from build123d import *

# Parameters (mm, degrees)
SKETCH1_W           = 113.157
SKETCH1_H           = 113.157
SKETCH1_R           = 3.048
BOSS_EXTRUDE1_DEPTH = 8.73125
SKETCH1_3_W         = 113.157
SKETCH1_3_H         = 113.157
SKETCH1_3_R         = 3.33375
SKETCH1_3_R_2       = 50.8
SKETCH1_3_R_3       = 3.01625
SKETCH1_3_R_4       = 3.048
BOSS_EXTRUDE2_DEPTH = 9.525
SKETCH1_4_R         = 3.01625
BOSS_EXTRUDE3_DEPTH = 18.3515
CUT_EXTRUDE1_START  = -5.899214
SKETCH2_R           = 3.5
CUT_EXTRUDE1_DEPTH  = 5.899214
CIRPATTERN1_COUNT   = 4
SKETCH5_R           = 3.047999999
BOSS_EXTRUDE4_DEPTH = 9.525


with BuildPart() as part:
    # Sketch1 → Boss-Extrude1 (new body)
    with BuildSketch(Plane.XY):
        Rectangle(SKETCH1_W, SKETCH1_H)
        with Locations((-14.204320599, -16.928050104)):
            Circle(SKETCH1_R, mode=Mode.SUBTRACT)
    extrude(amount=BOSS_EXTRUDE1_DEPTH)

    # Sketch1<3> → Boss-Extrude2 (add)
    with BuildSketch(Plane.XY):
        Rectangle(SKETCH1_3_W, SKETCH1_3_H)
        with Locations((-43.8785, -43.8785)):
            Circle(SKETCH1_3_R, mode=Mode.SUBTRACT)
        with Locations((43.8785, -43.8785)):
            Circle(SKETCH1_3_R, mode=Mode.SUBTRACT)
        with Locations((43.8785, 43.8785)):
            Circle(SKETCH1_3_R, mode=Mode.SUBTRACT)
        with Locations((-43.8785, 43.8785)):
            Circle(SKETCH1_3_R, mode=Mode.SUBTRACT)
        Circle(SKETCH1_3_R_2, mode=Mode.SUBTRACT)
        with Locations((24.490207929, 29.186293283)):
            Circle(SKETCH1_3_R_3)
        with Locations((13.030967461, -35.802288852)):
            Circle(SKETCH1_3_R_3)
        Circle(SKETCH1_3_R_3)
        with Locations((-37.52117539, 6.615995569)):
            Circle(SKETCH1_3_R_3)
        with Locations((-14.204320599, -16.928050104)):
            Circle(SKETCH1_3_R_4)
    extrude(amount=-BOSS_EXTRUDE2_DEPTH)

    # Sketch1<4> → Boss-Extrude3 (add)
    with BuildSketch(Plane.XY):
        Circle(SKETCH1_4_R)
    extrude(amount=-BOSS_EXTRUDE3_DEPTH)

    # Sketch2 → Cut-Extrude1 (cut)
    with BuildSketch(Plane(origin=(0, 56.5785, 0), x_dir=(1, 0, 0), z_dir=(0, 1, 0)).offset(CUT_EXTRUDE1_START)):
        with Locations((0, 4.7625)):
            Circle(SKETCH2_R)
    cut_extrude1 = extrude(amount=CUT_EXTRUDE1_DEPTH, mode=Mode.SUBTRACT)

    # CirPattern1: Cut-Extrude1 ×4 about axis
    cirpattern1_axis = Axis((0, 0, -9.525), (0, 0, 1))
    for i in range(1, CIRPATTERN1_COUNT):
        add(cut_extrude1.rotate(cirpattern1_axis, i * 360 / CIRPATTERN1_COUNT), mode=Mode.SUBTRACT)

    # Sketch5 → Boss-Extrude4 (add)
    with BuildSketch(Plane.XY.offset(8.73125)):
        with Locations((-14.204320599, -16.928050104)):
            Circle(SKETCH5_R)
    extrude(amount=-BOSS_EXTRUDE4_DEPTH)


solid = part.part
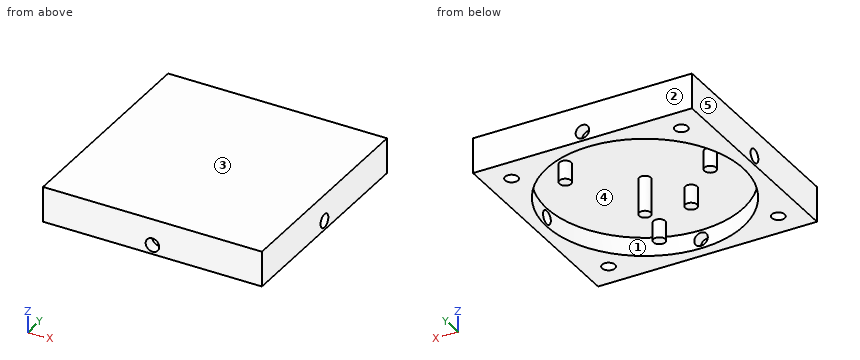
Input: part model. Units: mm. Frame: model coordinates. Face numbers are marked on the shaded views. A direction names the side the tool comes from. Give positions to 0.01 mm unless a question says otherwise; leave off trailing zeros. Order: outer loops, then holes, each group sorted by start corner. A loop starts at its lowest first (then second) coordinate and runs counter-clockwise, first axis right, second up. Notation, with made-up numbers: M -25,33.25 L 14,33.25 A22 ccw 14,40.25 Z; hole C 37.5,81 d9. An arc over 180 degrees is marked long. Answer as a JSON object with one key per item and string values.
1. Cut plane D-D, the plane y = 13.5. Output: boundary loops of the cut face in (x, z) (1 decimal).
Result sheet:
{"outline": "M -56.6,-9.5 L -49,-9.5 L -49,0 L 49,0 L 49,-9.5 L 56.6,-9.5 L 56.6,8.7 L -56.6,8.7 Z"}
2. First-contact query: P1, Ø4, axis at x = 0, z = -4.76, coming from the +Y side; P2, Ø7.5, axis at x = 45, y = -44.5, coming from the -Z side (3 decimals); P3, Ø5.5, axis at x = 43.88, y = 43.88, coming from the -Z side. Flat tips, straight axial feed; report the tip coordinate or a pass-through.
Result sheet:
{"P1": "y = 3.02", "P2": "z = -9.525", "P3": "z = 0"}
3. Ray query, line 1 (Z direction, x = 0, y = -53.35) (1 decimal); line 2 (Y direction, x = 14, z = -9); line 3 (Z direction, x = -8, y = 40). Return the intervals inside material, ascending. Write a range as [from, to].
Result sheet:
{"line 1": "[-9.5, -8.3], [-1.3, 8.7]", "line 2": "[-56.58, -48.83], [-38.66, -32.95], [48.83, 56.58]", "line 3": "[0, 8.73]"}
4. Reachability of the marked faces 1 and 2 from +Z, -Z, +X, -X, +Y, -Y: full face, straight path, thin tool, end or side. Return the list, or none.
Result sheet:
{"face 1": "-Z", "face 2": "+Z, -Z, +X, -X, +Y"}
5. Cut plane A-A, the plane x = 0. Output: boundary loops of the cut face in (y, z) (1 decimal), and give its area (3 significant figures).
Result sheet:
{"outline": "M -56.6,-9.5 L -50.8,-9.5 L -50.8,-8.3 L -56.6,-8.3 Z; M -56.6,-1.3 L -50.8,-1.3 L -50.8,0 L -3,0 L -3,-18.4 L 3,-18.4 L 3,0 L 50.8,0 L 50.8,-1.3 L 56.6,-1.3 L 56.6,8.7 L -56.6,8.7 Z; M 50.8,-9.5 L 56.6,-9.5 L 56.6,-8.3 L 50.8,-8.3 Z", "area": "1,130 mm²"}
6. Cut plane C-C, the plane x = -27.5. Output: boundary loops of the cut face in (y, z) (1 decimal), and give its area (3 significant figures).
Result sheet:
{"outline": "M -56.6,-9.5 L -42.7,-9.5 L -42.7,0 L 42.7,0 L 42.7,-9.5 L 56.6,-9.5 L 56.6,8.7 L -56.6,8.7 Z", "area": "1,250 mm²"}
7. Pull-direction query (X, two-part tool) for the marked faces 3, 4 and 5; classes: +X half, -X half, draft (parallel to the pull), parting line (faces both ways), or undercut.
Result sheet:
{"face 3": "draft", "face 4": "undercut", "face 5": "-X half"}
